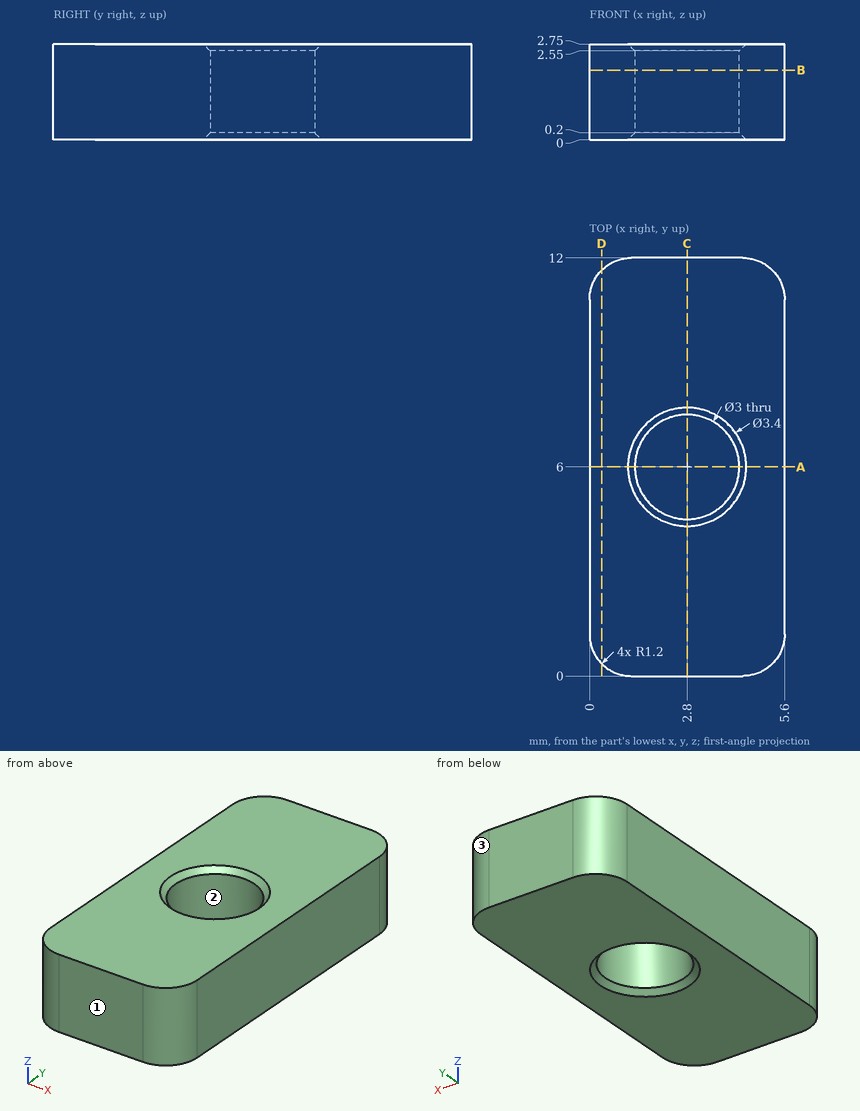
Could you check a few things on this drawing? It's one solid part, dimensions in mm from its lowest x, y, z. Give positions to 0.01 mm unless a question says otherwise; leave off trailing zeros. Write each loop counter-clockwise with the first axis right and the second up, starting at its lowest first coordinate (ties: lowest second). Pieces come first, ordered by that corner, then holes. Notation, with made-up numbers: (23, 39) -> (39, 39) arc R18 cw to (39, 59) -> close; hole circle Ø1 at (-2.5, 31). An arc over 180 degrees is marked (long way). Write item = value, one per line.
(1) I'm going to push flat-ended pins straight in: P1, Ø1, axis at x = 0.5, z = 1, coming from the -Y side; P2, Ø1, axis at x = 1, y = 7, coming from the -Z side. Where does each tip first touch, or does it pass through?
Worked out:
P1 = 0.02
P2 = 0
(2) Suppose I cut it at C-C on x = 2.8. Write out the boundary of the cut face in (y, z).
Worked out:
outline = (0, 0) -> (4.3, 0) -> (4.5, 0.2) -> (4.5, 2.55) -> (4.3, 2.75) -> (0, 2.75) -> close; (7.5, 0.2) -> (7.7, 0) -> (12, 0) -> (12, 2.75) -> (7.7, 2.75) -> (7.5, 2.55) -> close
(3) I need wall thicknesses on probe 1 along Y at (x, z) = (2.8, 1.65); probe 2 along Y at (x, z) = (4.45, 0.9); probe 3 along Y at (x, z) = (3.4, 1.75). Which ranges of each line are inside material? Lowest first, please. Write a range as from..to.
Worked out:
probe_1 = 0..4.5, 7.5..12
probe_2 = 0..12
probe_3 = 0..4.63, 7.37..12
(4) Thinking about a two-plate mould opening in Y: for the marked faces 1, 2 and 3, which applies, released by +Y, released by -Y, zero draft, split by the parting line, or undercut?
Worked out:
face_1 = released by -Y
face_2 = undercut
face_3 = released by +Y
(5) Suppose I cut it at D-D on x = 0.35. Write out the boundary of the cut face in (y, z), then the cut area to 3 significant figures.
Worked out:
outline = (0.35, 0) -> (11.65, 0) -> (11.65, 2.75) -> (0.35, 2.75) -> close
area = 31.1 mm^2
(6) Suppose I cut it at B-B on z = 2. Write out the boundary of the cut face in (x, y).
Worked out:
outline = (0, 1.2) arc R1.2 ccw to (1.2, 0) -> (4.4, 0) arc R1.2 ccw to (5.6, 1.2) -> (5.6, 10.8) arc R1.2 ccw to (4.4, 12) -> (1.2, 12) arc R1.2 ccw to (0, 10.8) -> close; hole circle Ø3 at (2.8, 6)
(7) Suppose I cut it at A-A on y = 6. Write out the boundary of the cut face in (x, z), then the cut area to 3 significant figures.
Worked out:
outline = (0, 0) -> (1.1, 0) -> (1.3, 0.2) -> (1.3, 2.55) -> (1.1, 2.75) -> (0, 2.75) -> close; (4.3, 0.2) -> (4.5, 0) -> (5.6, 0) -> (5.6, 2.75) -> (4.5, 2.75) -> (4.3, 2.55) -> close
area = 7.07 mm^2
